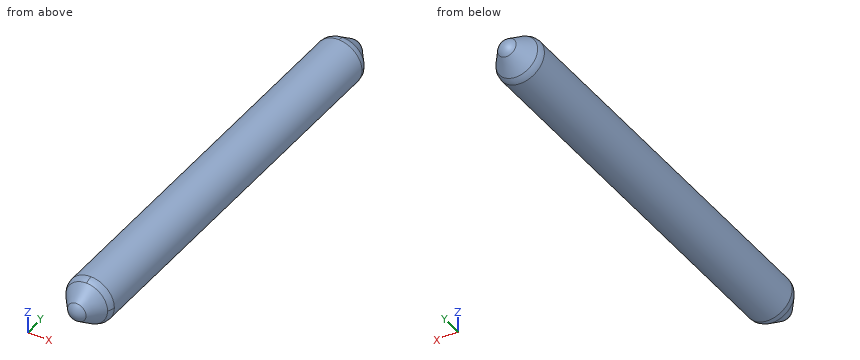
from build123d import *

# Parameters (mm, degrees)
SKETCH1_R           = 20
BOSS_EXTRUDE1_DEPTH = 170
FILLET1_R           = 10


with BuildPart() as part:
    # Sketch1 → Boss-Extrude1 (new, symmetric)
    with BuildSketch(Plane(origin=(0, 0, 0), x_dir=(-1, 0, 0), z_dir=(0, 1, 0))):
        with Locations(Location((0, 0, 0), (0, 0, 90))):
            Circle(SKETCH1_R)
    extrude(amount=BOSS_EXTRUDE1_DEPTH, both=True)

    # Sketch2 → Revolve1 (revolve)
    with BuildSketch(Plane(origin=(0, 0, 0), x_dir=(0, 1, 0), z_dir=(0, 0, 1)), mode=Mode.PRIVATE) as revolve1_sk:
        with BuildLine():
            Line((-170, 20), (-186, 8))
            ThreePointArc((-186, 8), (-188.94427191, 4.472135955), (-190, 0))
            Line((-190, 0), (-180, 0))
            Line((-180, 0), (-170, 0))
            Line((-170, 0), (-170, 20))
        make_face()
    revolve1 = revolve(revolve1_sk.sketch.rotate(Axis((0, -190, 0), (0, 1, 0)), 180), axis=Axis((0, -190, 0), (0, 1, 0)))

    # Mirror2: Revolve1 across plane
    add(revolve1.mirror(Plane.ZX))

    # Fillet1
    fillet1_edges = [part.edges().sort_by_distance(p)[0] for p in [
        (14.142135624, 170, 14.142135624),
        (-14.142135624, -170, -14.142135624),
    ]]
    fillet(fillet1_edges, radius=FILLET1_R)


solid = part.part
Verification items for the finished model (mm, model axes). Give positions to 0.01 mm unless a question says otherwise; leave off trailing zeros. Loops run counter-clockwise (first coordinate to the right, second up) from the corner with the lowest first, then second, coordinate; pieces in that order, holes last. Notation, with made-up numbers: (88.25, 3) - (136.25, 3) arc R14 cw to (136.25, 23) - close; hole circle Ø9 at (-39.75, 50.5). An arc over 180 degrees is marked (long way). Write item = value, one per line. Start each with the question number.
Q1. Depth check by flat-ended pin: P1, Ø12, axis at y = 55.5, z = 11, coming from the +X side; P2, Ø10, axis at x = 8, z = 11, coming from the +Y side; P3, Ø5, axis at x = -15.5, z = 10, coming from the +Y side. Enter the tip coordinate at first touch or a pass-through.
Q2. Cross-section at A-A, the plane y = 76. Enter the section's corners in (x, z).
Q3. Thickness scan on line 1 (Y direction, x = -0.5, z = 8); line 2 (Z direction, x = -4, y = 82.5); line 3 (X direction, y = 16, z = 14.5). Record the ranges inside material, lowest first.
Answer key:
q1.P1 = 19.36
q1.P2 = 185.2
q1.P3 = 175.41
q2.outline = circle Ø40 at (0, 0)
q3.line_1 = -185.98 to 185.98
q3.line_2 = -19.6 to 19.6
q3.line_3 = -13.77 to 13.77
